Verification items for this drawing (mm, ordinates from the low corner). A direction names the side the tool comes from. Round coordinates to 2 decimals unless told otherwise and drop trailing zeros. Write each loop counter-clockwise with the first axis right and the second up, starting at its lowest first coordinate (ties: lowest second). Pieces come first, ordered by that corner, then holes.
Item 1: Access from +Z, -Z, +X, -X, +Y, -Y to the whole of each face (thin tool, end or side, straight path). Record for the marked faces 1 and 2.
Item 2: Depth check by flat-ended pin: P1, Ø3, axis at y = 5, z = 7.5, coming from the -X side; P2, Ø5, axis at x = 3.5, z = 3.5, coming from the +Y side; P3, Ø4, axis at y = 5, z = 19, coming from the -X side; P4, Ø0.6, axis at x = 15.5, z = 16, coming from the -Y side. Enter the tip coordinate at first touch or a pass-through.
Item 3: Cross-section at C-C (y = 5). State how many separate pieces and enclosed holes the cut face has, then the cut area to 3 significant figures.
Item 4: Draft check along Y on the marked faces 3, 4 and 5. Enter one of: pulls with the +Y half, pulls with the -Y half, needs draft (parallel to the pull), parting line crosses it, or undercut.
Item 5: Scan lines: probe 1 along Z at (x, y) = (9.45, 5); probe 2 along X at (y, z) = (9, 4.5); probe 3 along X at (y, z) = (22, 23.75). Record each from-to range of solid material in increasing order.
Item 6: Cross-section at A-A (y = 9). Enter the section's corners in (x, z).
Item 7: Cross-section at B-B (z = 7.5). Enter the section's corners in (x, y), then the cut area to 3 significant figures.
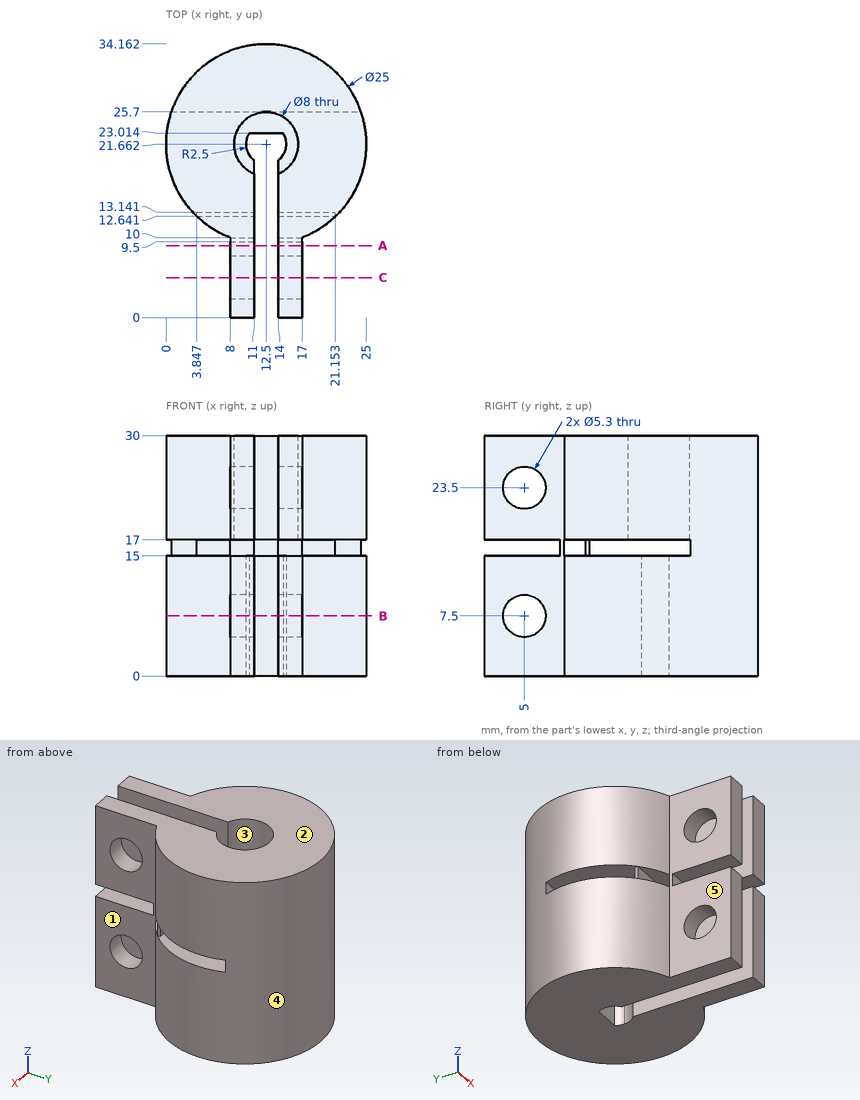
Resolved:
1. face 1: +Z, -Z, +X, -Y
1. face 2: +Z, +X, -X, +Y, -Y
2. P1: passes through
2. P2: stops at y = 32.34
2. P3: stops at x = 8
2. P4: stops at y = 9.5
3. separate pieces: 8
3. enclosed holes: 0
3. area: 104 mm2
4. face 3: undercut
4. face 4: parting line crosses it
4. face 5: needs draft
5. probe 1: z = 0 to 4.85, 10.15 to 15, 17 to 20.85, 26.15 to 30
5. probe 2: x = 8 to 11, 14 to 17
5. probe 3: x = 0 to 8.51, 16.49 to 25
6. outline: (8, 0) - (11, 0) - (11, 15) - (8, 15) - close; (8, 17) - (11, 17) - (11, 30) - (8, 30) - close; (14, 0) - (17, 0) - (17, 15) - (14, 15) - close; (14, 17) - (17, 17) - (17, 30) - (14, 30) - close
7. outline: (8, 0) - (11, 0) - (11, 2.35) - (8, 2.35) - close; (8, 7.65) - (11, 7.65) - (11, 19.66) arc R2.5 cw to (10.4, 23.01) - (14.6, 23.01) arc R2.5 cw to (14, 19.66) - (14, 7.65) - (17, 7.65) - (17, 10) arc R12.5 ccw (long way) to (8, 10) - close; (14, 0) - (17, 0) - (17, 2.35) - (14, 2.35) - close
7. area: 470 mm2
